```python
from build123d import *

# Parameters (mm, degrees)
F4_DEPTH = 30.001
F5_W     = 6
F5_H     = 7
F6_DEPTH = 13
F8_W     = 10
F8_H     = 4
F9_DEPTH = 7


with BuildPart() as f1:
    # F0 (on Right) → F1 (revolve)
    with BuildSketch(Plane.YZ):
        with BuildLine():
            Line((-30, 0), (0, 0))
            ThreePointArc((0, 0), (-15, 15), (-30, 0))
        make_face()
    revolve(axis=Axis((0, -15, 0), (0, -1, 0)))

    # F3 (on offset) → F4 (cut, through all)
    with BuildSketch(Plane.XY.offset(15)):
        with BuildLine():
            Line((15, 0), (0, 0))
            Line((0, 0), (-15, 0))
            ThreePointArc((-15, 0), (0, -3), (15, 0))
        make_face()
    extrude(amount=-F4_DEPTH, mode=Mode.SUBTRACT)

    # F5 (on Front) → F6 (cut)
    with BuildSketch(Plane.XZ):
        Rectangle(F5_W, F5_H)
    extrude(amount=F6_DEPTH, mode=Mode.SUBTRACT)

    # F8 (on offset) → F9 (cut)
    with BuildSketch(Plane.XY.offset(18)):
        with Locations((0, -15)):
            Rectangle(F8_W, F8_H)
        Polygon((-5, -17), (-5, -13), (-5, -10), (-10, -15), (-5, -20), align=None)
        Polygon((5, -10), (5, -13), (5, -17), (5, -20), (10, -15), align=None)
    extrude(amount=-F9_DEPTH, mode=Mode.SUBTRACT)


solid = f1.part
```
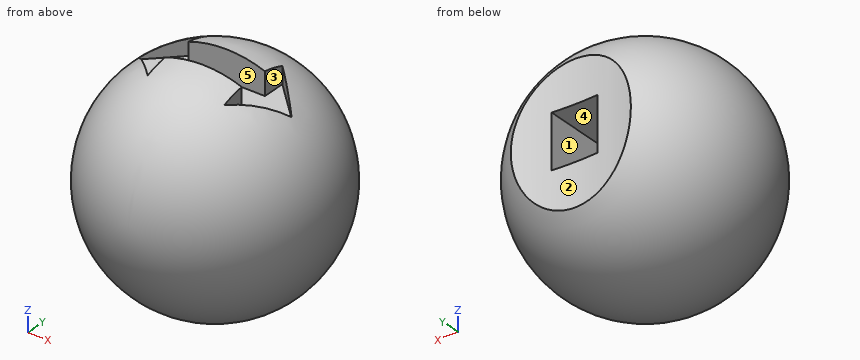
Geometry: final body of the model. Coordinates: model frame, mm. Face numbers are marked on the shaded views. A direction names the side the tool comes from. Round coordinates to 2 decimals unless told otherwise and drop trailing zeros. Write each loop counter-clockwise with the first axis right and the second up, starting at its lowest first coordinate (ties: lowest second). Pieces come first, ordered by that corner, then holes. Notation, with made-up numbers: (82.5, 11) -> (120.5, 11) arc R20 cw to (120.5, 23) -> close; hole circle Ø1 at (-35.5, 3.25). An arc over 180 degrees is marked (long way). Use CSV: the item, a comma, the result in double quotes. Start each with the question number.
Q1. Section B-B (y = -10.5). Return loops of the section in (x, z).
Q2. Section D-D (y = -28). Return loops of the section in (x, z).
Q3. Section A-A (z = 12.25). Return loops of the section in (x, y), plus the area to 3 significant figures.
Q4. Pull-direction query (Y, two-part tool) for the marked faces 1, 2 and 3; classes: pulls with the +Y half, pulls with the -Y half, needs draft (parallel to the pull), parting line crosses it, or undercut.
Q5. Section C-C (x = -2.5). Return loops of the section in (y, z), plus the area to 3 significant figures.
Q6. Reachability of the marked faces 4 and 5 from +Z, -Z, +X, -X, +Y, -Y: full face, straight path, thin tool, end or side. Return the list, or none.
Q7. First-contact query: pin 1 Ø3 at (x, y) = (-0.5, -9.5) entering from -Z; pin 2 Ø2 at (y, z) = (-9, 1) entering from +X; pin 3 Ø10 at (x, z) = (-2, 5) entering from +Y. Flat tips, straight axial feed; report the tip coordinate or a pass-through.
Q8. Line query: L1, parallel to Y at x = 1, z = 13.75; L2, parallel to Z at x = 1.25, y = -12.75; L3, parallel to Z at x = -1.5, y = -7. Output: solid intervals per line, ascending.
Result sheet:
1,outline,"(-5.5, 11) -> (-5.5, 13.21) arc R14.31 ccw (long way) to (5.5, 13.21) -> (5.5, 11) -> (5, 11) -> (5, 13.41) arc R14.31 ccw to (-5, 13.41) -> (-5, 11) -> close; hole (-3, -3.5) -> (3, -3.5) -> (3, 3.5) -> (-3, 3.5) -> close"
2,outline,"circle Ø14.97 at (0, 0)"
3,outline,"(-8.53, -16.47) arc R8.66 ccw to (8.53, -16.47) -> (5, -20) -> (5, -17) -> (-5, -17) -> (-5, -20) -> close; (-8.53, -13.53) -> (-5, -10) -> (-5, -13) -> (5, -13) -> (5, -10) -> (8.53, -13.53) arc R8.66 ccw to start"
3,area,"149 mm²"
4,face 1,"needs draft"
4,face 2,"pulls with the +Y half"
4,face 3,"undercut"
5,outline,"(-17, 11) -> (-17, 14.65) arc R14.79 ccw (long way) to (-2.92, -8.53) -> (-2.92, -3.5) -> (-13, -3.5) -> (-13, 3.5) -> (-2.92, 3.5) -> (-2.92, 8.53) arc R14.79 ccw to (-13, 14.65) -> (-13, 11) -> close"
5,area,"570 mm²"
6,face 4,"+Y"
6,face 5,"+Z"
7,pin 1,"z = -14.45"
7,pin 2,"x = 14.11"
7,pin 3,"y = -2.38"
8,L1,"-20.91 to -17, -13 to -9.09"
8,L2,"-14.78 to -3.5, 3.5 to 14.78"
8,L3,"-12.6 to -3.5, 3.5 to 12.6"
